```python
from build123d import *

# Parameters (mm, degrees)
F0_W     = 9.771576
F0_H     = 6.858
F1_DEPTH = 14.986
F2_W     = 9.906
F2_H     = 11.938
F3_DEPTH = 12.446
F4_R     = 1
F5_DEPTH = 2
F6_R     = 1
F8_DEPTH = 9.906


with BuildPart() as f1:
    # F0 (on Front) → F1 (new body)
    with BuildSketch(Plane.XZ):
        with BuildLine():
            ThreePointArc((4.885788, 3.429), (0, 5.969), (-4.885788, 3.429))
            Line((-4.885788, 3.429), (4.885788, 3.429))
        make_face()
        Rectangle(F0_W, F0_H)
        with BuildLine():
            Line((4.885788, -3.429), (-4.885788, -3.429))
            ThreePointArc((-4.885788, -3.429), (0, -5.969), (4.885788, -3.429))
        make_face()
    extrude(amount=F1_DEPTH)

    # F2 (on face) → F3 (join)
    with BuildSketch(Plane.XZ.offset(14.986)):
        Rectangle(F2_W, F2_H)
    extrude(amount=F3_DEPTH)

    # F4 (on face) → F5 (cut)
    with BuildSketch(Plane.XZ.offset(27.432)):
        with Locations((0, -4.572)):
            Circle(F4_R)
        with Locations((0, 4.572)):
            Circle(F4_R)
    extrude(amount=-F5_DEPTH, mode=Mode.SUBTRACT)

    # F6
    f6_edges = [f1.edges().sort_by_distance(p)[0] for p in [
        (-4.953, -21.209, 5.969),
        (4.953, -21.209, 5.969),
        (4.953, -21.209, -5.969),
        (-4.953, -21.209, -5.969),
    ]]
    fillet(f6_edges, radius=F6_R)

    # F7 (on face) → F8 (join)
    with BuildSketch(Plane.XZ.offset(27.432)):
        with BuildLine():
            ThreePointArc((-0.835155, 1.246), (-0.70614, -1.323392), (1.5, 0))
            ThreePointArc((1.5, 0), (1.323392, 0.70614), (0.835155, 1.246))
            Line((0.835155, 1.246), (-0.835155, 1.246))
        make_face()
    extrude(amount=F8_DEPTH)


solid = f1.part
```
The listing builds one solid part. Answer for the finished solid, in the listing's coordinates (mm). A direction names the side the tool comes from. Give positions to 0.01 mm unless a question says otherwise; leave off trailing zeros. Order: outer loops, then holes, each group sorted by start corner. A loop starts at its lowest first (then second) coordinate and runs counter-clockwise, first axis right, second up. Notation, with made-up numbers: (25.25, 82.25) -> (52.25, 82.25) arc R37 cw to (52.25, 119.25) -> close; hole circle Ø8 at (43.5, -22.5). An arc over 180 degrees is marked (long way). Answer as CSV lines item,"result". Start each with the question number.
Q1. Which of the six approach directions +Z, -Z, +X, -X, +Y, -Y give full straight-line access (tool end or side, diameter ignored) to faces 1 (the flat face through (-4.886, -7, 0)), 2 (the cylindrical face through (0.08, -7.39, 5.97)), 3 (the flat face through (0, -25.432, -5)), 4 (the cylindrical face through (-0.08, -7.39, -5.97))?
Q2. Given pin 1 (1.3 mm diameter, centred on x = 0, y = -31.5, fed in from +Z); pin 2 (5.5 mm diameter, centred on y = -10, z = 0, fed in from +X); pin 3 (1.6 mm diameter, centred on x = 0, z = 4.572, fed in from +Y); pin 4 (2 mm diameter, centred on x = -0.5, z = 5, fed in from -Y), each flat-ended and moving along its own axis, determine where each tip first touches the part or whether it passes through.
Q3. Determine the mould class of faces 5 (the flat face through (0, -32, 1.246)), 6 (the cylindrical face through (-4.668, -21.296, -5.668)), 7 (the flat face through (0, -25.432, 5)), 8 (the flat face through (4.886, -7, 0)) for opening direction X: pulls with the +X half, pulls with the -X half, needs draft (parallel to the pull), parting line crosses it, or undercut.
Q4. A cutting plane is placed at D-D (y = -33). Determine the outline of the cut face in (x, z), then the cut area to 3 significant figures.
Q5. A cutting plane is placed at A-A (y = -26). Determine the outline of the cut face in (x, z), then the cut area to 3 significant figures.
Q6. Find the intervals of material crossed by L1, parallel to Z at x = 0, y = -26.5; L2, parallel to Y at x = -2.25, z = 5.75; L3, parallel to Y at x = -0.75, z = -5.5, in increasing order.
Q7. A cutting plane is placed at B-B (z = -3). Determine the outline of the cut face in (x, y).
Q8. A cutting plane is placed at C-C (x = 2). Determine the outline of the cut face in (y, z), then the cut area to 3 significant figures.
Results found:
1,face 1,"+Z, -Z, -X, +Y"
1,face 2,"+Z, +Y"
1,face 3,"-Y"
1,face 4,"-Z, +Y"
2,pin 1,"z = 1.25"
2,pin 2,"x = 4.89"
2,pin 3,"y = 0"
2,pin 4,"y = -27.43"
3,face 5,"needs draft"
3,face 6,"pulls with the -X half"
3,face 7,"undercut"
3,face 8,"pulls with the +X half"
4,outline,"(-0.84, 1.25) arc R1.5 ccw (long way) to (0.84, 1.25) -> close"
4,area,"6.78 mm2"
5,outline,"(-4.95, -4.97) arc R1 ccw to (-3.95, -5.97) -> (3.95, -5.97) arc R1 ccw to (4.95, -4.97) -> (4.95, 4.97) arc R1 ccw to (3.95, 5.97) -> (-3.95, 5.97) arc R1 ccw to (-4.95, 4.97) -> close; hole circle Ø2 at (0, -4.57); hole circle Ø2 at (0, 4.57)"
5,area,"111 mm2"
6,L1,"-5.97 to -5.57, -3.57 to 3.57, 5.57 to 5.97"
6,L2,"-27.43 to -14.99"
6,L3,"-27.43 to 0"
7,outline,"(-4.95, -27.43) -> (4.95, -27.43) -> (4.95, -14.99) -> (4.89, -14.99) -> (4.89, 0) -> (-4.89, 0) -> (-4.89, -14.99) -> (-4.95, -14.99) -> close"
8,outline,"(-27.43, -5.97) -> (-14.99, -5.97) -> (-14.99, -5.62) -> (0, -5.62) -> (0, 5.62) -> (-14.99, 5.62) -> (-14.99, 5.97) -> (-27.43, 5.97) -> close"
8,area,"317 mm2"
